The figure shows three views and two pictorial views of one solid part (mm, origin at its lowest corner). Answer the questions. A direction names the side the tool comes from. Round coordinates to 2 decimals unless told otherwise and drop trailing zeros. Write each loop counter-clockwise with the first axis right and the second up, starting at its lowest first coordinate (ties: lowest second). Pieces come first, ordered by that corner, then holes. Notation, with made-up numbers: (-23.5, 2.25) - (-10.5, 2.25) arc R8 ccw to (-10.5, 16.25) - close; hole circle Ø1 at (-19.75, 84.25). An arc over 180 degrees is marked (long way). Answer as CSV lines item,"result". Start each with the question number.
Item 1: For a pull along Y with two mould halves and no side action, classify the marked faces 4, 5, 6 and 7 as pulls with the +Y half, pulls with the -Y half, needs draft (parallel to the pull), parting line crosses it, or undercut.
Item 2: Flat-ended cylindrical pins translate along their axes: pin 1 (8 mm diameter, centred on y = 27, z = 6, fed in from +X); pin 2 (4.5 mm diameter, centred on x = 23.5, y = 11.5, fed in from +Z); pin 3 (2 mm diameter, centred on x = 56, y = 38.5, fed in from -Z); pin 4 (3 mm diameter, centred on y = 16.5, z = 2.5, fed in from +X). Find the tip coordinate at first contact, or state that the pin passes through.
Item 3: Straight lines are drawn through the part: line 1 along Y through (x, z) = (23.5, 4); line 2 along X through (y, z) = (66.5, 5.5); line 3 along Y through (x, z) = (21.5, 10). For each, find the intervals that lie inside material, in ascending order. Write a range as [from, to].
Item 4: A cutting plane is placed at D-D on y = 66.5. Determine the outline of the cut face in (x, z), and give its area (3 significant figures).
Item 5: Which of the six approach directions +Z, -Z, +X, -X, +Y, -Y give full straight-line access (tool end or side, diameter ignored) to the marked faces 1, 2 and 3?
Item 6: A cutting plane is placed at B-B on z = 17.75. Determine the outline of the cut face in (x, y).
Item 7: A cutting plane is placed at C-C on x = 39. Determine the outline of the cut face in (y, z), and give its area (3 significant figures).
Item 8: A cutting plane is placed at A-A on y = 40.5. Determine the outline of the cut face in (x, z), and give its area (3 significant figures).
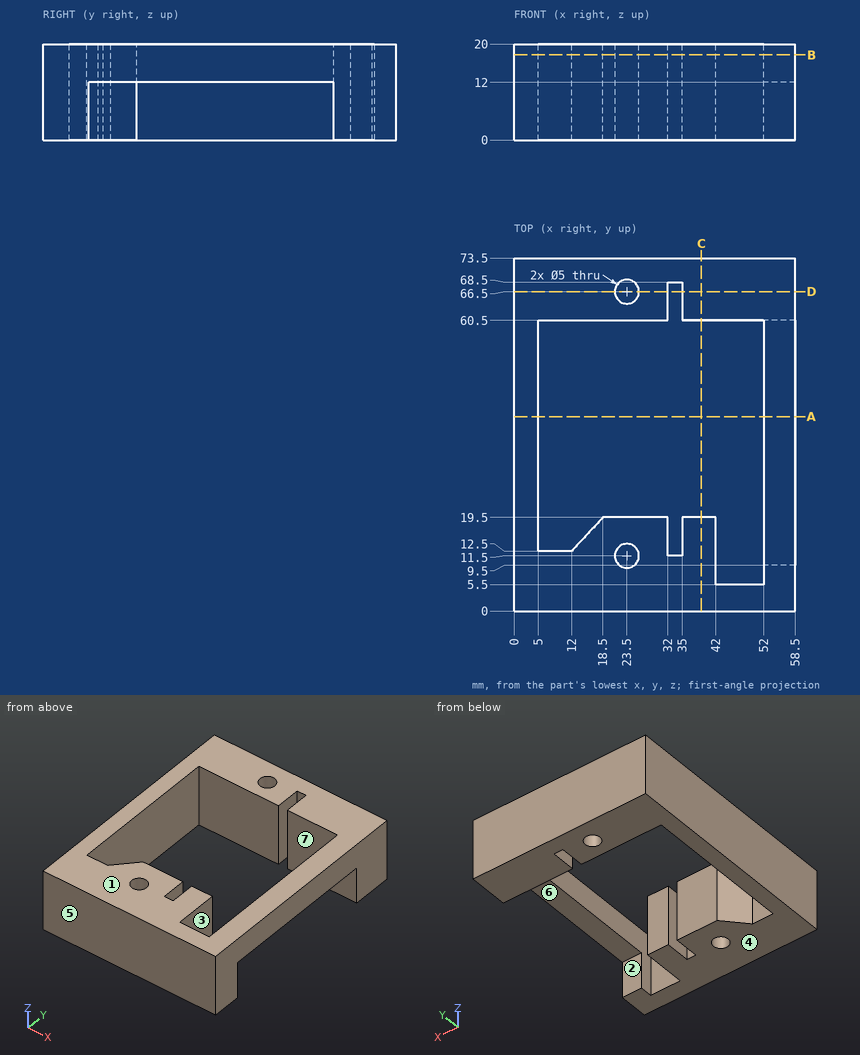
Geometry says:
1,face 4,"needs draft"
1,face 5,"pulls with the -Y half"
1,face 6,"undercut"
1,face 7,"undercut"
2,pin 1,"stops at x = 5"
2,pin 2,"passes through"
2,pin 3,"stops at z = 12"
2,pin 4,"stops at x = 42"
3,line 1,"y = [0, 9], [14, 19.5], [60.5, 64], [69, 73.5]"
3,line 2,"x = [0, 21], [26, 32], [35, 58.5]"
3,line 3,"y = [0, 10], [13, 19.5], [60.5, 65], [68, 73.5]"
4,outline,"(0, 0) - (21, 0) - (21, 20) - (0, 20) - close; (26, 0) - (32, 0) - (32, 20) - (26, 20) - close; (35, 0) - (58.5, 0) - (58.5, 20) - (35, 20) - close"
4,area,"1,010 mm^2"
5,face 1,"+Z, +X, -X, +Y, -Y"
5,face 2,"-Z, +X"
5,face 3,"+Z, -Z"
6,outline,"(0, 0) - (58.5, 0) - (58.5, 73.5) - (0, 73.5) - close; hole (5, 12.5) - (12, 12.5) - (18.5, 19.5) - (32, 19.5) - (32, 11.5) - (35, 11.5) - (35, 19.5) - (42, 19.5) - (42, 5.5) - (52, 5.5) - (52, 60.5) - (35, 60.5) - (35, 68.5) - (32, 68.5) - (32, 60.5) - (5, 60.5) - close; hole circle Ø5 at (23.5, 11.5); hole circle Ø5 at (23.5, 66.5)"
7,outline,"(0, 0) - (19.5, 0) - (19.5, 20) - (0, 20) - close; (60.5, 0) - (73.5, 0) - (73.5, 20) - (60.5, 20) - close"
7,area,"650 mm^2"
8,outline,"(0, 0) - (5, 0) - (5, 20) - (0, 20) - close; (52, 12) - (58.5, 12) - (58.5, 20) - (52, 20) - close"
8,area,"152 mm^2"
